Source: three-view drawing plus pictorial views. Frame: mm from the lowest corner of the part. A direction names the side the tool comes from. Round coordinates to 2 decimals unless told otherwise and drop trailing zeros. Loops run counter-clockwise (first coordinate to the right, second up) from the corner with the lowest first, then second, coordinate; pieces in that order, holes last. Notation, with made-up numbers: (-27, 33) -> (10, 33) arc R17 ccw to (10, 50) -> close; hole circle Ø3 at (15.25, 64.25). An arc over 180 degrees is marked (long way). Answer in a Markdown table with one row per item.
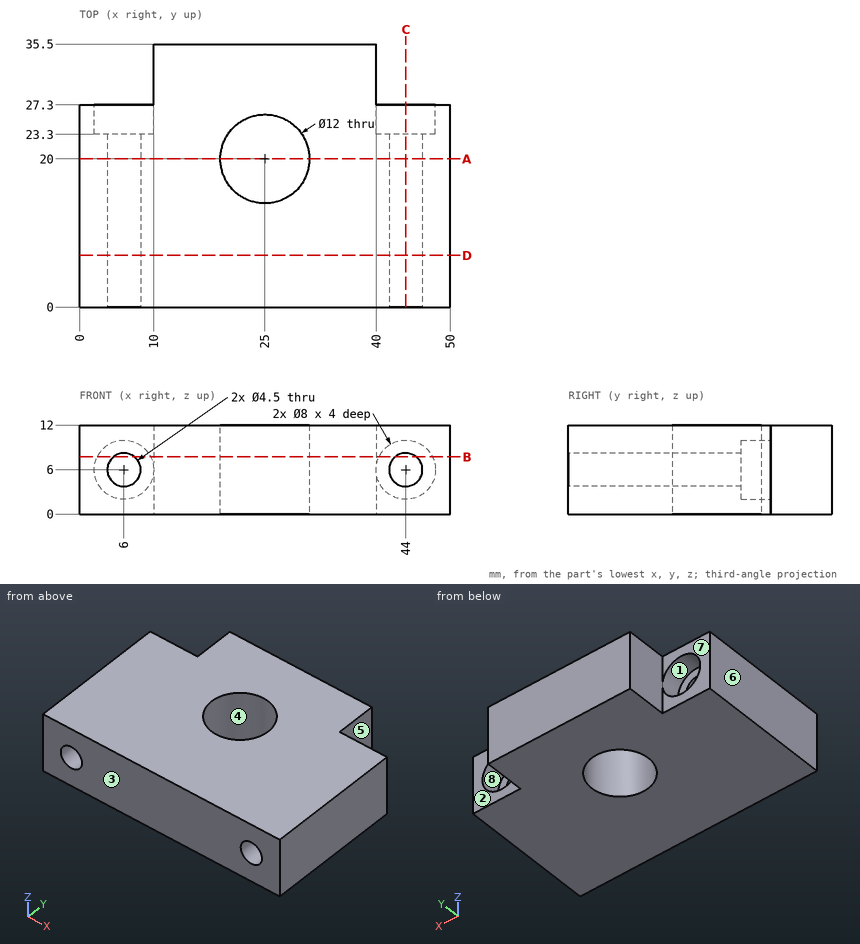
Item 1: Cut plane A-A (y = 20). Output: boundary loops of the cut face in (x, z).
Answer:
| item | result |
|---|---|
| outline | (0, 0) -> (19, 0) -> (19, 12) -> (0, 12) -> close; (31, 0) -> (50, 0) -> (50, 12) -> (31, 12) -> close; hole circle Ø4.5 at (6, 6); hole circle Ø4.5 at (44, 6) |
Item 2: Cut plane D-D (y = 7). Output: boundary loops of the cut face in (x, z), then the cut area to 3 significant figures.
Answer:
| item | result |
|---|---|
| outline | (0, 0) -> (50, 0) -> (50, 12) -> (0, 12) -> close; hole circle Ø4.5 at (6, 6); hole circle Ø4.5 at (44, 6) |
| area | 568 mm² |
Item 3: Draft query along Y for the marked faces 1, 2, 3 and 4. Return one class per face: pulls with the +Y half, pulls with the -Y half, needs draft (parallel to the pull), parting line crosses it, or undercut.
Answer:
| item | result |
|---|---|
| face 1 | needs draft |
| face 2 | pulls with the +Y half |
| face 3 | pulls with the -Y half |
| face 4 | undercut |
Item 4: Cut plane C-C (x = 44). Output: boundary loops of the cut face in (y, z), then the cut area to 3 significant figures.
Answer:
| item | result |
|---|---|
| outline | (0, 0) -> (27.3, 0) -> (27.3, 2) -> (23.3, 2) -> (23.3, 3.75) -> (0, 3.75) -> close; (0, 8.25) -> (23.3, 8.25) -> (23.3, 10) -> (27.3, 10) -> (27.3, 12) -> (0, 12) -> close |
| area | 191 mm² |
Item 5: Line query: probe 1 along Z at (x, y) = (6, 5); probe 2 along Z at (x, y) = (6, 24.5); probe 3 along X at (y, z) = (10, 4). Output: solid intervals per line, ascending. Write a range as [from, to].
Answer:
| item | result |
|---|---|
| probe 1 | z = [0, 3.75], [8.25, 12] |
| probe 2 | z = [0, 2], [10, 12] |
| probe 3 | x = [0, 4.97], [7.03, 42.97], [45.03, 50] |
Item 6: Reachability of the marked faces 5, 6, 7 and 8 from +Z, -Z, +X, -X, +Y, -Y: full face, straight path, thin tool, end or side. Return the list, or none.
Answer:
| item | result |
|---|---|
| face 5 | +Z, -Z, +X, +Y |
| face 6 | +Z, -Z, -X, +Y, -Y |
| face 7 | +Z, -Z, -X, +Y |
| face 8 | +Y |
Item 7: Cut plane B-B (z = 7.75). Output: boundary loops of the cut face in (x, y).
Answer:
| item | result |
|---|---|
| outline | (0, 0) -> (4.59, 0) -> (4.59, 23.3) -> (2.4, 23.3) -> (2.4, 27.3) -> (0, 27.3) -> close; (7.41, 0) -> (42.59, 0) -> (42.59, 23.3) -> (40.4, 23.3) -> (40.4, 27.3) -> (40, 27.3) -> (40, 35.5) -> (10, 35.5) -> (10, 27.3) -> (9.6, 27.3) -> (9.6, 23.3) -> (7.41, 23.3) -> close; (45.41, 0) -> (50, 0) -> (50, 27.3) -> (47.6, 27.3) -> (47.6, 23.3) -> (45.41, 23.3) -> close; hole circle Ø12 at (25, 20) |
Item 8: Pin query (flat end, axial travel): pin 1 Ø2.5 at (y, z) = (32.5, 4) entering from -X; pin 2 Ø3.5 at (x, z) = (44, 6) entering from -Y; pin 3 Ø5 at (x, z) = (5, 6) entering from +Y. Return the tip coordinate at first contact, or that it passes through.
Answer:
| item | result |
|---|---|
| pin 1 | stops at x = 10 |
| pin 2 | passes through |
| pin 3 | stops at y = 23.3 |
